Geometry: final body of the model. Coordinates: model frame, mm. Round coordinates to 2 decimals unless told otherwise and drop trailing zeros. Order: outer loops, then holes, each group sorted by start corner. A loop starts at its lowest first (then second) coordinate and runs counter-clockwise, first axis right, second up. Notation, with made-up numbers: (44, 72.5) -> (55, 72.5) arc R17 ccw to (55, 103.5) -> close; hole circle Ø11 at (-31, 84). An arc over 180 degrees is marked (long way). Put each result on its own line as item: value.
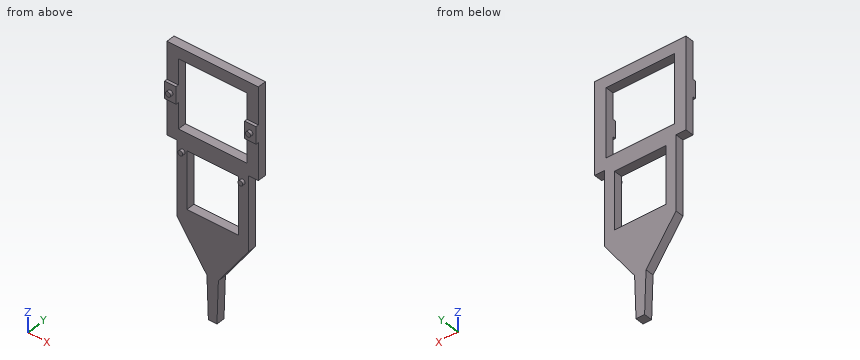
```python
from build123d import *

# Parameters (mm, degrees)
F0_R     = 0.9
F1_DEPTH = 5
F0_R_2   = 0.85
F2_DEPTH = 4
F0_W     = 4
F0_H     = 6
F3_DEPTH = 4
F4_DEPTH = 3
F5_DEPTH = 3


# Not quite as in the source:
# - a feature names something its author has since deleted; it is built from what else it names


with BuildPart() as f1:
    # F0 (on Front) → F1 (new body)
    with BuildSketch(Plane.XZ):
        with Locations((-14, 12)):
            Circle(F0_R)
    extrude(amount=F1_DEPTH)

    # F0 (on Front) → F3 (join)
    with BuildSketch(Plane.XZ):
        with Locations((-14, 12)):
            Rectangle(F0_W, F0_H)
        with Locations((-14, 12)):
            Circle(F0_R, mode=Mode.SUBTRACT)
    extrude(amount=F3_DEPTH)



with BuildPart() as f1b:
    # F0 (on Front) → F1, piece 2 (new body)
    with BuildSketch(Plane.XZ):
        with Locations((14, 12)):
            Circle(F0_R)
    extrude(amount=F1_DEPTH)

    # F0 (on Front) → F3, piece 2 (join)
    with BuildSketch(Plane.XZ):
        with Locations((14, 12)):
            Rectangle(F0_W, F0_H)
        with Locations((14, 12)):
            Circle(F0_R, mode=Mode.SUBTRACT)
    extrude(amount=F3_DEPTH)


with BuildPart() as f2:
    # F0 (on Front) → F2 (new body)
    with BuildSketch(Plane.XZ):
        with Locations((-10.5, -7)):
            Circle(F0_R_2)
    extrude(amount=F2_DEPTH)


with BuildPart() as f2b:
    # F0 (on Front) → F2, piece 2 (new body)
    with BuildSketch(Plane.XZ):
        with Locations((10.5, -7)):
            Circle(F0_R_2)
    extrude(amount=F2_DEPTH)


with BuildPart() as f1_1:
    add(f1.part)

    add(f1b.part)  # F4 merges F1b

    add(f2.part)  # F4 merges F2

    add(f2b.part)  # F4 merges F2b
    # F0 (on Front) → F4 (join)
    with BuildSketch(Plane.XZ):
        Polygon((-12, 24), (0, 24), (0, 28), (-16, 28), (-16, 15), (-12, 15), align=None)
        Polygon((0, 28), (0, 24), (12, 24), (12, 15), (16, 15), (16, 28), align=None)
        Polygon((0, 0), (0, -4), (12.5, -4), (16, -4), (16, 9), (12, 9), (12, 0), align=None)
        Polygon((-16, -4), (-12.5, -4), (0, -4), (0, 0), (-12, 0), (-12, 9), (-16, 9), align=None)
        Polygon((0, -4), (-12.5, -4), (-12.5, -30), (0, -30), (0, -26), (-9, -26), (-9, -6), (0, -6), align=None)
        with Locations((-10.5, -7)):
            Circle(F0_R_2, mode=Mode.SUBTRACT)
        Polygon((12.5, -4), (0, -4), (0, -6), (9, -6), (9, -26), (0, -26), (0, -30), (12.5, -30), align=None)
        with Locations((10.5, -7)):
            Circle(F0_R_2, mode=Mode.SUBTRACT)
    extrude(amount=F4_DEPTH)

    # F0 (on Front) → F5 (join)
    with BuildSketch(Plane.XZ):
        Polygon((0, -30), (-12.5, -30), (-2, -45), (2, -45), (12.5, -30), align=None)
        Polygon((2, -45), (-2, -45), (-1.5, -60), (1.5, -60), align=None)
    extrude(amount=F5_DEPTH)


solid = f1_1.part
```
1. Cut plane A-A on z = 12. Return loops of the section in (x, y).
Ans:
outline: (-16, -4) -> (-14.9, -4) -> (-14.9, -5) -> (-13.1, -5) -> (-13.1, -4) -> (-12, -4) -> (-12, 0) -> (-16, 0) -> close; (12, -4) -> (13.1, -4) -> (13.1, -5) -> (14.9, -5) -> (14.9, -4) -> (16, -4) -> (16, 0) -> (12, 0) -> close
2. Cut plane B-B on x = 5.5. Return loops of the section in (y, z).
Ans:
outline: (-3, -40) -> (0, -40) -> (0, -26) -> (-3, -26) -> close; (-3, -6) -> (0, -6) -> (0, 0) -> (-3, 0) -> close; (-3, 24) -> (0, 24) -> (0, 28) -> (-3, 28) -> close
3. Contact query for flat-ended pins moving along their axis: P1, Ø1.1, axis at x = -14, y = -3.5, coming from the +Z side; P2, Ø0.5, axis at x = 10, z = -7, coming from the -Y side; P3, Ø14.5, axis at x = -5.5, z = 20.5, coming from the -Y side; P4, Ø1.5, axis at y = -4, z = -6.5, coming from the +X side. Output: stop coordinate, or through.
Ans:
P1: z = 28
P2: y = -4
P3: y = -3
P4: x = 11.35
4. Cut plane C-C on y = -1.1. Return loops of the section in (x, z).
Ans:
outline: (-16, -4) -> (-12.5, -4) -> (-12.5, -30) -> (-2, -45) -> (-1.5, -60) -> (1.5, -60) -> (2, -45) -> (12.5, -30) -> (12.5, -4) -> (16, -4) -> (16, 28) -> (-16, 28) -> close; hole (-12, 0) -> (12, 0) -> (12, 24) -> (-12, 24) -> close; hole (-9, -26) -> (9, -26) -> (9, -6) -> (-9, -6) -> close
5. Cut plane D-D on x = 10.5. Return loops of the section in (y, z).
Ans:
outline: (-4, -7.85) -> (-3, -7.85) -> (-3, -32.86) -> (0, -32.86) -> (0, 0) -> (-3, 0) -> (-3, -6.15) -> (-4, -6.15) -> close; (-3, 24) -> (0, 24) -> (0, 28) -> (-3, 28) -> close
6. Material intervals for probe 1 along X at (y, z) = (-3.4, 11.5); probe 2 along X at (y, z) = (-1.5, -7); probe 3 along Z at (x, y) = (-5, -1.6), sorted ascending.
Ans:
probe 1: -16 to -12, 12 to 16
probe 2: -12.5 to -9, 9 to 12.5
probe 3: -40.71 to -26, -6 to 0, 24 to 28
